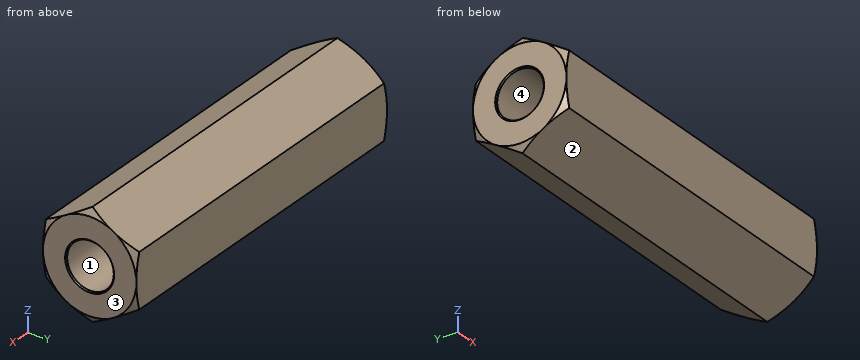
from build123d import *

# Parameters (mm, degrees)
BOSS_EXTRUDE1_DEPTH = 30
SKETCH4_OUTSIDE_W   = 125.104
SKETCH4_OUTSIDE_H   = 123.866
SKETCH4_OUTSIDE_R   = 4
CUT_EXTRUDE1_DEPTH  = 31
CUT_EXTRUDE1_TAPER  = 60
SKETCH5_OUTSIDE_W   = 125.104
SKETCH5_OUTSIDE_H   = 123.866
SKETCH5_OUTSIDE_R   = 4
CUT_EXTRUDE2_DEPTH  = 31
CUT_EXTRUDE2_TAPER  = 60


with BuildPart() as part:
    # Sketch2 → Boss-Extrude1 (new body)
    with BuildSketch(Plane(origin=(0, 0, 0), x_dir=(0, 0, -1), z_dir=(1, 0, 0))):
        Polygon((2.309401077, 4), (-2.309401077, 4), (-4.618802154, 0), (-2.309401077, -4), (2.309401077, -4), (4.618802154, 0), align=None)
    extrude(amount=BOSS_EXTRUDE1_DEPTH)

    # Sketch3 → Cut-Revolve1 (revolve, cut)
    with BuildSketch(Plane.XY):
        Polygon((0, 2.1), (0.1, 2), (11.1, 2), (11.1, 0), (0, 0), align=None)
        Polygon((30, 0), (18.9, 0), (18.9, 2), (29.9, 2), (30, 2.1), align=None)
    revolve(axis=Axis((0, 0, 0), (1, 0, 0)), mode=Mode.SUBTRACT)

    # Sketch4 outside → Cut-Extrude1 (cut, through all)
    with BuildSketch(Plane.ZY):
        Rectangle(SKETCH4_OUTSIDE_W, SKETCH4_OUTSIDE_H)
        Circle(SKETCH4_OUTSIDE_R, mode=Mode.SUBTRACT)
    extrude(amount=-CUT_EXTRUDE1_DEPTH, taper=CUT_EXTRUDE1_TAPER, mode=Mode.SUBTRACT)

    # Sketch5 outside → Cut-Extrude2 (cut, through all)
    with BuildSketch(Plane(origin=(30, 0, 0), x_dir=(0, 0, -1), z_dir=(1, 0, 0))):
        Rectangle(SKETCH5_OUTSIDE_W, SKETCH5_OUTSIDE_H)
        Circle(SKETCH5_OUTSIDE_R, mode=Mode.SUBTRACT)
    extrude(amount=-CUT_EXTRUDE2_DEPTH, taper=CUT_EXTRUDE2_TAPER, mode=Mode.SUBTRACT)


solid = part.part
Here's how the part is built. I have some questions about the finished solid (model axes, mm). Face numbers are marked on the shaded views. Coordinates: 2 decimals unless noted, no trailing zeros. Loops run counter-clockwise (first coordinate to the right, second up) from the corner with the lowest first, then second, coordinate; pieces in that order, holes last.
1. Imagine slicing it at A-A, the plane x = 28. Please give me the cut outline in (y, z), and give its area (3 significant figures).
2. Imagine slicing it at B-B, the plane x = 17. Please give me the cut outline in (y, z).
3. I need wall thicknesses on L1, parallel to X at y = 0.25, z = 0; L2, parallel to Z at x = 24.25, y = 0.75; L3, parallel to Z at x = 2, y = 0.25. Which ranges of each line are inside material? Lowest first, please.
4. For P1, Ø1, axis at x = 19, y = 1.5, coming from the -Z side; P2, Ø3.5, axis at y = 0, z = 0, coming from the -X side, each with a flat end and sliding along its axis, tell me the tip position at first contact or that it passes through.
5. If we mould it in two halves opening along Z, with no side actions, what happens to the marked faces 1, 2, 3 and 4? For each: pulls with the +Z half, pulls with the -Z half, needs draft (parallel to the pull), parting line crosses it, or undercut.
Taken from the geometry:
1. outline: (-4, -2.31) - (0, -4.62) - (4, -2.31) - (4, 2.31) - (0, 4.62) - (-4, 2.31) - close; hole circle Ø4 at (0, 0)
1. area: 42.9 mm2
2. outline: (-4, -2.31) - (0, -4.62) - (4, -2.31) - (4, 2.31) - (0, 4.62) - (-4, 2.31) - close
3. L1: x = 11.1 to 18.9
3. L2: z = -4.19 to -1.85, 1.85 to 4.19
3. L3: z = -4.47 to -1.98, 1.98 to 4.47
4. P1: stops at z = -4.04
4. P2: stops at x = 11.1
5. face 1: undercut
5. face 2: pulls with the -Z half
5. face 3: needs draft
5. face 4: undercut
